Autodesk Inventor part; units mm, degrees
ref_plane "YZ Plane" through (0, 0, 0) normal (1, 0, 0) x (0, 1, 0)
ref_plane "XZ Plane" through (0, 0, 0) normal (0, 1, 0) x (-1, 0, 0)
ref_plane "XY Plane" through (0, 0, 0) normal (0, 0, 1) x (1, 0, 0)
sketch "Sketch1" plane through (0, 0, 0) normal (0, 0, 1) x (1, 0, 0)
  line L0 (-6.5, 0) -> (6.5, 0) construction
  line L1 (-6.5, -2) -> (6.5, -2)
  line L2 (6.5, 2) -> (-6.5, 2)
  arc A0 (-6.5, 2) -> (-6.5, -2) centre (-6.5, 0) ccw
  arc A1 (6.5, -2) -> (6.5, 2) centre (6.5, 0) ccw
  point P0 (0, 0)
  dimension "d0" = 17
  dimension "d1" = 4
extrude "Extrusion1" add sketch "Sketch1" along normal blind 5
sketch "Sketch2" plane through (0, 0, 5) normal (0, 0, 1) x (1, 0, 0)
  circle A0 centre (0, 0) radius 6
  dimension "d4" = 12
extrude "Extrusion2" cut sketch "Sketch2" against normal blind 0.75
sketch "Sketch3" plane through (0, 0, 4.25) normal (0, 0, 1) x (1, 0, 0)
  circle A0 centre (0, 0) radius 1
  dimension "d7" = 2
extrude "Extrusion3" add sketch "Sketch3" along normal blind 0.5
hole "Hole1" at (0, 0, 4.75) direction (0, 0, -1) diameter 1.2 depth 3.3 tip angle 118
sketch "Sketch4" plane through (0, 0, 0) normal (0, 0, -1) x (-1, 0, 0)
  line L0 (6.5, -2) -> (-6.5, -2)
  arc A0 (6.5, -2) -> (6.5, 2) centre (6.5, 0) ccw
  line L1 (-6.5, 2) -> (6.5, 2)
  arc A1 (-6.5, 2) -> (-6.5, -2) centre (-6.5, 0) ccw
  line L2 (-4.5, 2) -> (4.5, 2) construction
  line L3 (-6.5, 2) -> (6.5, 2)
  line L4 (-4.5, 1.5) -> (4.5, 1.5)
  line L5 (4.5, 2.5) -> (-4.5, 2.5)
  arc A2 (-4.5, 2.5) -> (-4.5, 1.5) centre (-4.5, 2) ccw
  arc A3 (4.5, 1.5) -> (4.5, 2.5) centre (4.5, 2) ccw
  point P0 (0, 0)
  point P1 (0, 2)
  point P2 (0, 2)
  dimension "d19" = 0.5
  dimension "d20" = 10
extrude "Extrusion4" cut sketch "Sketch4" against normal through all contours A3 L4 A2 L1 | L1 A2 L5 A3
properties part number "phalanx_1_gearbox_support"
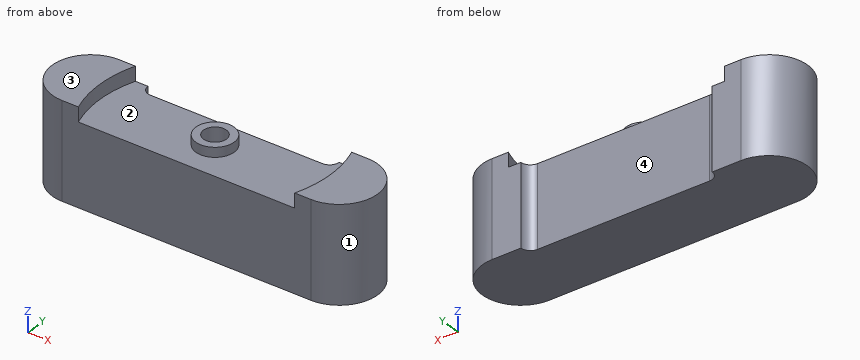
Check sheet for the modelled part. Datum: model origin and axes. Units: mm. Face numbers are marked on the shaded views. Coordinates: 2 decimals unless noted, no trailing zeros. Order: outer loops, then holes, each group sorted by start corner. A loop starts at its lowest first (then second) coordinate and runs counter-clockwise, first axis right, second up. Notation, with made-up numbers: M -35.75,39 L -4.75,39 A18 cw -4.75,51 Z; hole C 46.25,-30.5 d11. An arc over 180 degrees is marked long. One line per question, with ' | ' between items. Start each with the question number.
Item 1: Sectioned sample at B-B on y = -1.6. Record the cut outline in (x, z), and give its area (3 significant figures).
Item 2: Gauge pin test, flat ends, axial feed: P1, Ø1, axis at x = 0.5, z = 2.5, coming from the +Y side; P2, Ø1, axis at x = 0, y = 0.5, coming from the +Z side; P3, Ø1.5, axis at y = 1, z = 4, coming from the +X side. Record the tip position at first contact, or that the pin passes through.
Item 3: Sectioned sample at D-D on x = 3.5. Record the cut outline in (y, z), and give its area (3 significant figures).
Item 4: Material ranges on line 1 (X direction, y = 0, z = 2.4); line 2 (Y direction, x = 0, z = 3.45); line 3 (Z direction, x = -1.5, y = -1.8), recorded low to high.
Item 5: Mould release check, pull along X, two halves, no side actions. Record for the marked faces 1, 2, 3 and 4: pulls with the +X half, pulls with the -X half, needs draft (parallel to the pull), parting line crosses it, or undercut.
Item 6: Sectioned sample at A-A on z = 2.7. Record the cut outline in (x, y), and give its area (3 significant figures).
Item 7: Sectioned sample at C-C on x = 0.75. Record the cut outline in (y, z).
Answer below:
1) outline: M -7.7,0 L 7.7,0 L 7.7,5 L 5.78,5 L 5.78,4.25 L -5.78,4.25 L -5.78,5 L -7.7,5 Z | area: 68.3 mm^2
2) P1: stops at y = 1.5 | P2: stops at z = 4.75 | P3: stops at x = 8.48
3) outline: M -2,0 L 1.5,0 L 1.5,4.25 L -2,4.25 Z | area: 14.9 mm^2
4) line 1: x = -8.5 to -0.6, 0.6 to 8.5 | line 2: y = -2 to -0.6, 0.6 to 1.5 | line 3: z = 0 to 4.25
5) face 1: pulls with the +X half | face 2: undercut | face 3: needs draft | face 4: undercut
6) outline: M -6.5,-2 L 6.5,-2 A2 ccw 6.5,2 L 5,2 A0.5 cw 4.5,1.5 L -4.5,1.5 A0.5 cw -5,2 L -6.5,2 A2 ccw Z; hole C 0,0 d1.2 | area: 58.5 mm^2
7) outline: M -2,0 L 1.5,0 L 1.5,4.25 L 0.66,4.25 L 0.66,4.75 L -0.66,4.75 L -0.66,4.25 L -2,4.25 Z
